```python
from build123d import *

# Parameters (mm, degrees)
EXTRUDE_1_DEPTH     = 15
SKETCH_2_R          = 2.5
CUT_EXTRUDE_1_DEPTH = 589.461978381
SKETCH_2_3_R        = 2.5
CUT_EXTRUDE_2_DEPTH = 589.461978381
SKETCH_4_R          = 2.5
CUT_EXTRUDE_3_DEPTH = 589.461978381


with BuildPart() as part:
    # ｽｹｯﾁ1 → ﾎﾞｽ - 押し出し1 (new body)
    with BuildSketch(Plane.XY):
        Polygon((-242.5, 297.5), (242.5, 297.5), (507.5, -297.5), (-242.5, -297.5), align=None)
    extrude(amount=EXTRUDE_1_DEPTH)

    # ｽｹｯﾁ2 → ｶｯﾄ - 押し出し1 (cut, through all)
    with BuildSketch(Plane.XY.offset(15)):
        with Locations((-192.5, 287.5)):
            Circle(SKETCH_2_R)
        with Locations((2.5, 287.5)):
            Circle(SKETCH_2_R)
        with Locations((197.5, 287.5)):
            Circle(SKETCH_2_R)
    cut_extrude_1 = extrude(amount=-CUT_EXTRUDE_1_DEPTH, mode=Mode.SUBTRACT)

    # ｽｹｯﾁ2<3> → ｶｯﾄ - 押し出し2 (cut, through all)
    with BuildSketch(Plane.XY.offset(15)):
        with Locations((-232.5, 247.5)):
            Circle(SKETCH_2_3_R)
        with Locations((-232.5, 0)):
            Circle(SKETCH_2_3_R)
        with Locations((-232.5, -247.5)):
            Circle(SKETCH_2_3_R)
    cut_extrude_2 = extrude(amount=-CUT_EXTRUDE_2_DEPTH, mode=Mode.SUBTRACT)

    # ﾐﾗｰ1: ｶｯﾄ - 押し出し1 across plane
    add(cut_extrude_1.mirror(Plane.ZX), mode=Mode.SUBTRACT)

    # ﾐﾗｰ2: ｶｯﾄ - 押し出し2 across plane
    add(cut_extrude_2.mirror(Plane(origin=(0, 0, 0), x_dir=(0, 0, 1), z_dir=(1, 0, 0))), mode=Mode.SUBTRACT)

    # ｽｹｯﾁ4 → ｶｯﾄ - 押し出し3 (cut, through all)
    with BuildSketch(Plane.XY.offset(15)):
        with Locations((372.5, -287.5)):
            Circle(SKETCH_4_R)
    extrude(amount=-CUT_EXTRUDE_3_DEPTH, mode=Mode.SUBTRACT)


solid = part.part
```
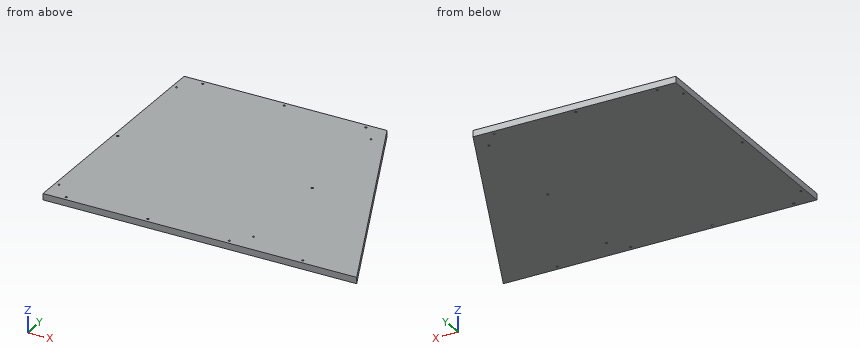
Here's how the part is built. I have some questions about the finished solid (model axes, mm). Round coordinates to 2 decimals unless told otherwise and drop trailing zeros. Loops run counter-clockwise (first coordinate to the right, second up) from the corner with the lowest first, then second, coordinate; pieces in that order, holes last. Notation, with made-up numbers: (31.5, 31) -> (71.5, 31) arc R25 ccw to (71.5, 58) -> close; hole circle Ø7 at (37.5, -21.75). An arc over 180 degrees is marked (long way). Answer as CSV lines item,"result".
1. If we section it at C-C on x = 273.5: Please give me the cut outline in (y, z).
Final values:
outline,"(-297.5, 0) -> (227.9, 0) -> (227.9, 15) -> (-297.5, 15) -> close"
2. If we section it at B-B on y = -105.5: Please give me the cut outline in (x, z).
Final values:
outline,"(-242.5, 0) -> (421.99, 0) -> (421.99, 15) -> (-242.5, 15) -> close"
3. If I drill on L1, parallel to Y at x = 197.5, z = 5; L2, parallel to X at y = -287.5, z = 3.75; L3, parallel to X at y = -247.5, z = 9, over which ranges is the centre line in solid material (lowest first)?
Final values:
L1,"y = -297.5 to -290, -285 to 285, 290 to 297.5"
L2,"x = -242.5 to -195, -190 to 0, 5 to 195, 200 to 370, 375 to 503.05"
L3,"x = -242.5 to -235, -230 to 230, 235 to 485.23"
4. If we section it at A-A on z = 6: Count the separate pieces of the cut face and the enclosed holes in it, plus the area to 3 significant figures.
Final values:
separate pieces,"1"
enclosed holes,"13"
area,"367,000 mm^2"
5. For pin 1 (5 mm diameter, centred on y = 189, z = 10, fed in from +X); pin 2 (8 mm diameter, centred on y = -194, z = 8, fed in from +X); pin 3 (5 mm diameter, centred on y = 116, z = 5.5, fed in from +X), each with a flat end and sliding along its axis, tell me the tip position at first contact or that it passes through.
Final values:
pin 1,"stops at x = 291.94"
pin 2,"stops at x = 463.18"
pin 3,"stops at x = 324.45"
